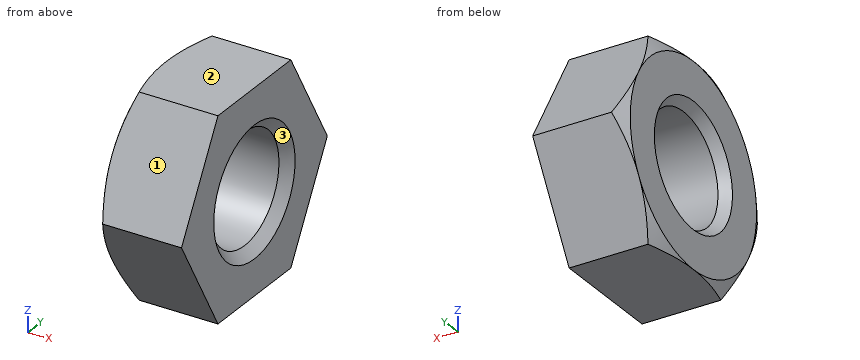
```python
from build123d import *

# Parameters (mm, degrees)
SKETCH3_W               = 11
SKETCH3_H               = 11
CUT_EXTRUDE1_DEPTH      = 1.2
CUT_EXTRUDE1_DEPTH_BACK = 1.2


with BuildPart() as part:
    # Sketch1 → Revolve1 (revolve)
    with BuildSketch(Plane.XY):
        Polygon((-1.2, 0), (-1.2, 2.75), (-0.940192379, 3.2), (1.2, 3.2), (1.2, 0), align=None)
    revolve(axis=Axis((1.2, 0, 0), (-1, 0, 0)))

    # Sketch2 → Cut-Revolve1 (revolve, cut)
    with BuildSketch(Plane.XY):
        Polygon((-1.2, 0), (-1.2, 1.7), (-0.9295, 1.5), (0.9295, 1.5), (1.2, 1.7705), (1.2, 0), align=None)
    revolve(axis=Axis((1.2, 0, 0), (-1, 0, 0)), mode=Mode.SUBTRACT)

    # Sketch3 → Cut-Extrude1 (cut, two sides)
    with BuildSketch(Plane(origin=(0, 0, 0), x_dir=(0, 0, -1), z_dir=(1, 0, 0))) as cut_extrude1_sk:
        Rectangle(SKETCH3_W, SKETCH3_H)
        Polygon((-2.75, -1.58771324), (0, -3.175426481), (2.75, -1.58771324), (2.75, 1.58771324), (0, 3.175426481), (-2.75, 1.58771324), align=None, mode=Mode.SUBTRACT)
    extrude(amount=CUT_EXTRUDE1_DEPTH, mode=Mode.SUBTRACT)
    extrude(cut_extrude1_sk.sketch, amount=-CUT_EXTRUDE1_DEPTH_BACK, mode=Mode.SUBTRACT)


solid = part.part
```
Design review of the part built by this model. Coordinates are the model's own, in mm. Face numbers are marked on the shaded views. Round coordinates to 2 decimals unless told otherwise and drop trailing zeros. Write each loop counter-clockwise with the first axis right and the second up, starting at its lowest first coordinate (ties: lowest second). Pieces come first, ordered by that corner, then holes. Notation, with made-up numbers: (87, 77.25) -> (110, 77.25) arc R33 cw to (110, 111.25) -> close; hole circle Ø10 at (-12.75, -6.75). An arc over 180 degrees is marked (long way). Write item = value, one per line. Start each with the question number.
1) Take a section at B-B, the plane x = 1. State the section outline as (y, z) points.
2) Mouldability with a two-part tool opening along Y and no side actions: class the marked faces 1, 2 and 3 as +Y half, -Y half, draft (parallel to the pull), parting line (faces both ways), or undercut.
3) Take a section at A-A, the plane x = 0.35. State the section outline as (y, z) points, plus the area to 3 significant figures.
4) Wall thickness on probe 1 along Z at (x, y) = (-0.2, 0); probe 2 along Y at (x, z) = (-0.8, 0.55); probe 3 along Y at (x, z) = (1.05, -0.45): over which ranges is each line inside the solid? List them lowest first. Write a range as from..to.
Results list:
q1.outline = (-3.18, 0) -> (-1.59, -2.75) -> (1.59, -2.75) -> (3.18, 0) -> (1.59, 2.75) -> (-1.59, 2.75) -> close; hole circle Ø3.14 at (0, 0)
q2.face_1 = -Y half
q2.face_2 = draft
q2.face_3 = undercut
q3.outline = (-3.18, 0) -> (-1.59, -2.75) -> (1.59, -2.75) -> (3.18, 0) -> (1.59, 2.75) -> (-1.59, 2.75) -> close; hole circle Ø3 at (0, 0)
q3.area = 19.1 mm²
q4.probe_1 = -2.75..-1.5, 1.5..2.75
q4.probe_2 = -2.86..-1.4, 1.4..2.86
q4.probe_3 = -2.92..-1.56, 1.56..2.92
